Design review of the part built by this model. Coordinates are the model's own, in mm. Coordinates: 2 decimals unless noted, no trailing zeros. Loops run counter-clockwise (first coordinate to the right, second up) from the corner with the lowest first, then second, coordinate; pieces in that order, holes last. Notation, with made-up numbers: M 69.5,40.5 L 77.5,40.5 A18 ccw 77.5,67.5 Z; hole C -9,65 d5. An arc over 180 degrees is marked long. One line per item, written item: value.
```python
from build123d import *

# Parameters (mm, degrees)
F0_R            = 172.5
F0_R_2          = 140
F1_DEPTH        = 3
F2_R            = 3
F3_DEPTH        = 25
F3_COPIES_COUNT = 11


# Not quite as in the source:
# - a pattern or mirror of a feature is missing from the dataset's text; its kind, count and spacing are read off the source's solid


with BuildPart() as f1:
    # F0 (on Front) → F1 (new body)
    with BuildSketch(Plane.XZ):
        Circle(F0_R)
        Circle(F0_R_2, mode=Mode.SUBTRACT)
    extrude(amount=F1_DEPTH)

    # F2 (on face) → F3 (cut)
    with BuildSketch(Plane.XZ.offset(3)):
        with Locations((0, 156.4114242792)):
            Circle(F2_R)
    f3 = extrude(amount=-F3_DEPTH, mode=Mode.SUBTRACT)

    # F3_copies: F3 ×11 about axis
    f3_copies_axis = Axis((0, 0, 0), (0, 1, 0))
    for i in range(1, F3_COPIES_COUNT):
        add(f3.rotate(f3_copies_axis, i * 360 / F3_COPIES_COUNT), mode=Mode.SUBTRACT)


solid = f1.part
```
(1) We need section C-C on y = -1.4. State how many separate pieces and enclosed holes the cut face has, then the cut area to 3 significant figures.
Reply:
separate pieces: 1
enclosed holes: 12
area: 31,600 mm2
(2) To check wall thickness, follow line 1 along Z through (x, y) = (0, -2.2); line 2 along X through (y, z) = (-2.35, -21); line 3 along X through (y, z) = (-1.95, -100). State the ranges of each line that lie inside material, in increasing order. Write a range as [from, to].
Reply:
line 1: z = [-172.5, -140], [140, 153.41], [159.41, 172.5]
line 2: x = [-171.22, -157.54], [-152.1, -138.42], [138.42, 152.1], [157.54, 171.22]
line 3: x = [-140.56, -119.97], [-116.45, -97.98], [97.98, 116.45], [119.97, 140.56]
(3) Insertion check: pin 1 (5.5 mm diameter, centred on x = 142.28, z = 64.98, fed in from -Y); pin 2 (1.5 mm diameter, centred on x = 61, y = -1, fed in from -Z); pin 3 (1 mm diameter, centred on x = -107, y = -2.5, fed in from +Z). Each pin has a flat end and moves straight along its axis. Give the tip position at first contact, or say it passes through.
Reply:
pin 1: passes through
pin 2: stops at z = -161.64
pin 3: stops at z = 135.7
(4) We need section B-B on x = -52.5. State the section outline as (y, z) points, then the cut area to 3 significant figures.
Reply:
outline: M -3,-164.32 L 0,-164.32 L 0,-129.78 L -3,-129.78 Z; M -3,129.78 L 0,129.78 L 0,164.32 L -3,164.32 Z
area: 207 mm2
(5) We need section A-A on z = 0. State the section outline as (x, y) points, then the cut area to 3 significant figures.
Reply:
outline: M -172.5,-3 L -140,-3 L -140,0 L -172.5,0 Z; M 140,-3 L 172.5,-3 L 172.5,0 L 140,0 Z
area: 195 mm2
(6) Mouldability with a two-part tool opening along X and no side actions: class faces 1 (the cylindrical face through (164.534, -1.479, 51.814)), 2 (the flat face through (-1, 0, 141)), 3 (the cylindrical face through (-111.1, -1.48, -85.19)) as released by +X, released by -X, zero draft, split by the parting line, or undercut.
Reply:
face 1: split by the parting line
face 2: zero draft
face 3: undercut
